Geometry check sheet. Reference: the model listing, model coordinates, mm. A direction names the side the tool comes from. Round coordinates to 2 decimals unless told otherwise and drop trailing zeros. Write each loop counter-clockwise with the first axis right and the second up, starting at its lowest first coordinate (ties: lowest second). Pieces come first, ordered by that corner, then holes. Notation, with made-up numbers: M 66.5,60 L 125.5,60 A10 ccw 125.5,69 Z; hole C -5,2 d10. An arc over 180 degrees is marked long. Use a Markdown table: item, result.
Autodesk Inventor part; units mm, degrees
ref_plane "YZ Plane" through (0, 0, 0) normal (1, 0, 0) x (0, 1, 0)
ref_plane "XZ Plane" through (0, 0, 0) normal (0, 1, 0) x (-1, 0, 0)
ref_plane "XY Plane" through (0, 0, 0) normal (0, 0, 1) x (1, 0, 0)
sketch "Sketch1" plane through (0, 0, 0) normal (0, 0, 1) x (1, 0, 0)
  line L0 (0, 0) -> (0, 7.105)
  line L1 (0, 0) -> (0, -7.105)
  line L2 (0, -7.105) -> (-5, -7.105)
  line L3 (-5, -7.105) -> (-5, 7.105)
  line L4 (0, 7.105) -> (-5, 7.105)
  circle A0 centre (-2.5, -7.105) radius 2.5
  circle A1 centre (-2.5, 7.105) radius 2.5
  circle A2 centre (-2.5, -7.105) radius 1
  circle A3 centre (-2.5, 7.105) radius 1
  line L5 (-5, 0) -> (-5, 2.4)
  line L6 (-5, 2.4) -> (-25.5, 2.4)
  line L7 (-25.5, 2.4) -> (-25.5, -2.4)
  line L8 (-25.5, -2.4) -> (-5, -2.4)
  dimension "d0" = 7.105
  dimension "d1" = 7.105
  dimension "d2" = 5
  dimension "d3" = 5
  dimension "d4" = 5
  dimension "d5" = 2
  dimension "d6" = 2
  dimension "d7" = 2.4
  dimension "d8" = 20.5
  dimension "d9" = 4.8
extrude "Extrusion1" add sketch "Sketch1" against normal blind 2 contours L1 A0 L3 A1 L0 | A1 L4 A3 | L4 A3 A1 | A0 L2 A2 | L2 A2 A0 | L3 L8 L7 L6
sketch "Sketch2" plane through (0, 0, -2) normal (0, 0, -1) x (-1, 0, 0)
  line L0 (0, 7.105) -> (0, -7.105)
  arc A0 (0, -7.105) -> (5, -7.105) centre (2.5, -7.105) ccw
  line L1 (5, -7.105) -> (5, -2.4)
  line L2 (5, -2.4) -> (25.5, -2.4)
  line L3 (25.5, -2.4) -> (25.5, 2.4)
  line L4 (25.5, 2.4) -> (5, 2.4)
  line L5 (5, 2.4) -> (5, 7.105)
  arc A1 (5, 7.105) -> (0, 7.105) centre (2.5, 7.105) ccw
  circle A2 centre (2.5, -7.105) radius 1
  circle A3 centre (2.5, 7.105) radius 1
  line L6 (23, 2.4) -> (25.5, 2.4)
  line L7 (25.5, 2.4) -> (25.5, -2.4)
  line L8 (25.5, -2.4) -> (23, -2.4)
  line L9 (23, -2.4) -> (23, 2.4)
  point P0 (0, 0)
  point P1 (23, -2.4)
  dimension "d26" = 2.5
extrude "Extrusion2" add sketch "Sketch2" along normal blind 2.905 contours L4 L3 L2 L9
sketch "Sketch4" plane through (0, 0, 0) normal (0, 0, 1) x (1, 0, 0)
  arc A0 (0, 7.105) -> (-5, 7.105) centre (-2.5, 7.105) ccw
  line L0 (-5, 7.105) -> (-5, 2.4)
  line L1 (-5, 2.4) -> (-25.5, 2.4)
  line L2 (-25.5, 2.4) -> (-25.5, -2.4)
  line L3 (-25.5, -2.4) -> (-5, -2.4)
  line L4 (-5, -2.4) -> (-5, -7.105)
  arc A1 (-5, -7.105) -> (0, -7.105) centre (-2.5, -7.105) ccw
  line L5 (0, -7.105) -> (0, 7.105)
  circle A2 centre (-2.5, -7.105) radius 1
  circle A3 centre (-2.5, 7.105) radius 1
  line L6 (-25.5, 0) -> (-27.5, 0)
  circle A4 centre (-27.5, 0) radius 1.5
  circle A5 centre (-27.5, 0) radius 2.4
  line L7 (-25.5, -2.4) -> (-27.5, -2.4)
  line L8 (-25.5, 2.4) -> (-27.5, 2.4)
  point P0 (0, 0)
  dimension "d21" = 2
  dimension "d22" = 3
  dimension "d23" = 4.8
extrude "Extrusion4" add sketch "Sketch4" against normal up to surface (4.905 mm away) contours L2 A5 L8 | L2 A5 | L7 A5 L2 picked at (-25.6812, 0.5619)
mirror "Mirror2" about plane through (-24.25, 0, -4.905) normal (0, 0, -1) of "Extrusion1", "Extrusion2", "Extrusion4"
equation "\"d1\" = d0"
equation "\"d3\" = d2"
equation "\"d4\" = d2"
equation "\"d6\" = d5"
equation "\"d9\" = 2 * d7"
properties part number "PistonPivotTop"
Item 1: Material ranges on line 1 along Y through (x, z) = (-2.5, -8.7) (3 decimals); line 2 along Z through (x, y) = (-19.5, -0.25); line 3 along Y through (x, z) = (-15, -9.25), recorded low to high. Write a range as from..to.
Outcome:
| item | result |
|---|---|
| line 1 | y = -9.605..-8.105, -6.105..6.105, 8.105..9.605 |
| line 2 | z = -9.81..-7.81, -2..0 |
| line 3 | y = -2.4..2.4 |
Item 2: Cross-section at A-A, the plane y = -5.25. Record the cut outline in (x, z).
Outcome:
| item | result |
|---|---|
| outline | M -5,-9.81 L 0,-9.81 L 0,-7.81 L -5,-7.81 Z; M -5,-2 L 0,-2 L 0,0 L -5,0 Z |
Item 3: Access from +Z, -Z, +X, -X, +Y, -Y to the whole of each face (thin tool, end or side, straight path). Record for faces 1 (the face through (-5, 5, -9)), 2 (the face through (-9, 0, -7.81)), 3 (the face through (-5, -5, -9)).
Outcome:
| item | result |
|---|---|
| face 1 | +Z, -Z, -X, +Y |
| face 2 | +X, +Y, -Y |
| face 3 | +Z, -Z, -X, -Y |
Item 4: Go/stop test with flat-tipped pins: pin 1 (4 mm diameter, centred on y = -6, z = -2.5, fed in from -X); pin 2 (1.5 mm diameter, centred on x = -4.5, z = -8, fed in from +Y); pin 3 (2 mm diameter, centred on x = -5.5, z = -7.5, fed in from +Y). Record where each tip stops, or that it passes through.
Outcome:
| item | result |
|---|---|
| pin 1 | stops at x = -5 |
| pin 2 | stops at y = 9.27 |
| pin 3 | stops at y = 8.54 |
Item 5: Cross-section at B-B, the plane x = -9.5. Record the cut outline in (y, z).
Outcome:
| item | result |
|---|---|
| outline | M -2.4,-9.81 L 2.4,-9.81 L 2.4,-7.81 L -2.4,-7.81 Z; M -2.4,-2 L 2.4,-2 L 2.4,0 L -2.4,0 Z |
Item 6: Cross-section at C-C, the plane z = -0.75. Record the cut outline in (x, y) (3 decimals), and give its area (3 significant figures).
Outcome:
| item | result |
|---|---|
| outline | M -27.5,-2.4 L -5,-2.4 L -5,-7.105 A2.5 ccw 0,-7.105 L 0,7.105 A2.5 ccw -5,7.105 L -5,2.4 L -27.5,2.4 A2.4 ccw Z; hole C -27.5,0 d3; hole C -2.5,-7.105 d2; hole C -2.5,7.105 d2 |
| area | 194 mm2 |
Item 7: Cross-section at D-D, the plane x = -2.5. Record the cut outline in (y, z) (3 decimals).
Outcome:
| item | result |
|---|---|
| outline | M -9.605,-9.81 L -8.105,-9.81 L -8.105,-7.81 L -9.605,-7.81 Z; M -9.605,-2 L -8.105,-2 L -8.105,0 L -9.605,0 Z; M -6.105,-9.81 L 6.105,-9.81 L 6.105,-7.81 L -6.105,-7.81 Z; M -6.105,-2 L 6.105,-2 L 6.105,0 L -6.105,0 Z; M 8.105,-9.81 L 9.605,-9.81 L 9.605,-7.81 L 8.105,-7.81 Z; M 8.105,-2 L 9.605,-2 L 9.605,0 L 8.105,0 Z |
Item 8: Mould release check, pull along Y, two halves, no side actions. Record for faces 4 (the face through (-2.445, -9.604, -8.824)), 5 (the face through (-29.9, 0.05, -4.84)), 6 (the face through (-2.72, -8.08, -0.99)), 7 (the face through (0, 0, -9)): +Y half, -Y half, draft (parallel to the pull), parting line (faces both ways), or undercut.
Outcome:
| item | result |
|---|---|
| face 4 | -Y half |
| face 5 | parting line |
| face 6 | undercut |
| face 7 | draft |
